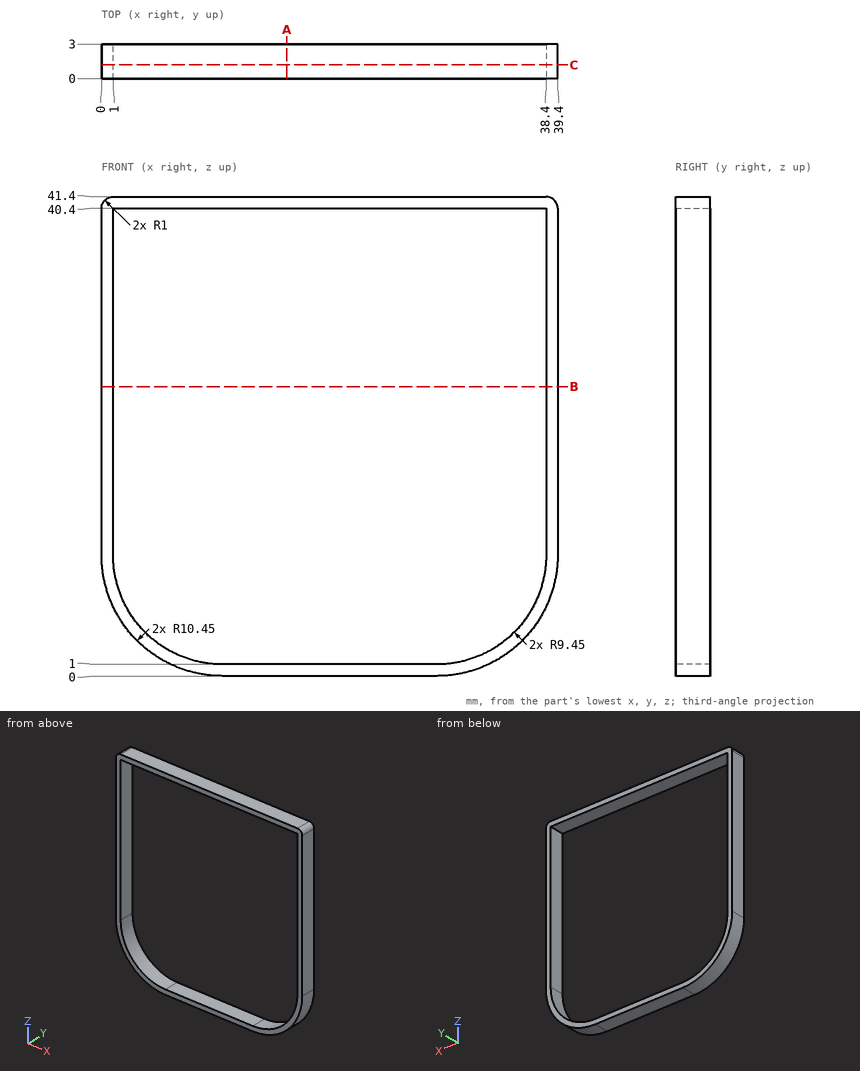
Design review of the part shown in the three views and the two pictorial views. Dimensions are in mm from the part's minimum x, y and z. Round coordinates to 2 decimals unless told otherwise and drop trailing zeros. Order: outer loops, then holes, each group sorted by start corner. A loop starts at its lowest first (then second) coordinate and runs counter-clockwise, first axis right, second up.
Q1. Wall thickness on line 1 (Z direction, x = 23.5, y = 2.55); line 2 (X direction, y = 0.85, z = 35.5); line 3 (Z direction, x = 36, y = 1.8): over which ranges is each line inside the solid? List them lowest first.
Findings below:
line 1: z = 0 to 1, 40.4 to 41.4
line 2: x = 0 to 1, 38.4 to 39.4
line 3: z = 2.74 to 4.16, 40.4 to 41.4
Q2. We need section A-A, the plane x = 16. Give the boundary of the cut face in (y, z), plus the area to 3 significant figures.
Findings below:
outline: (0, 0) - (3, 0) - (3, 1) - (0, 1) - close; (0, 40.4) - (3, 40.4) - (3, 41.4) - (0, 41.4) - close
area: 6.00 mm2
Q3. We need section B-B, the plane z = 25. Give the boundary of the cut face in (x, y).
Findings below:
outline: (0, 0) - (1, 0) - (1, 3) - (0, 3) - close; (38.4, 0) - (39.4, 0) - (39.4, 3) - (38.4, 3) - close
Q4. We need section C-C, the plane y = 1.2. Give the boundary of the cut face in (x, z).
Findings below:
outline: (0, 10.45) arc R10.45 ccw to (10.45, 0) - (28.95, 0) arc R10.45 ccw to (39.4, 10.45) - (39.4, 40.4) arc R1 ccw to (38.4, 41.4) - (1, 41.4) arc R1 ccw to (0, 40.4) - close; hole (1, 10.45) arc R9.45 ccw to (10.45, 1) - (28.95, 1) arc R9.45 ccw to (38.4, 10.45) - (38.4, 40.4) - (1, 40.4) - close
Q5. Insertion check: P1, Ø1, axis at x = 17, y = 2.5, coming from the -Z side. The pin has a flat end and moves straight along its axis. Give the tip position at first contact, or say it passes through.
Findings below:
P1: stops at z = 0
